from build123d import *

# Parameters (mm, degrees)
F0_R      = 8.89
F1_DEPTH  = 12.7
F2_R      = 6.35
F3_DEPTH  = 27.94
F5_DEPTH  = 43.18
F6_R      = 20.2522571076
F6_R_2    = 6.3246
F7_DEPTH  = 43.18
F8_R      = 4
F9_DEPTH  = 33.02
F13_D     = 2.2606
F13_DEPTH = 8.89
F13_START = 0.0721476
F13_TIP   = 0.6791527577
F14_R     = 8.89
F14_R_2   = 3.175
F15_DEPTH = 11.43


with BuildPart() as f1:
    # F0 (on Top) → F1 (new body)
    with BuildSketch(Plane.XY):
        Circle(F0_R)
    extrude(amount=F1_DEPTH)

    # F2 (on face) → F3 (join)
    with BuildSketch(Plane.XY.offset(12.7)):
        Circle(F2_R)
    extrude(amount=F3_DEPTH)

    # F4 (on face) → F5 (join)
    with BuildSketch(Plane.XY.offset(40.64)):
        Polygon((0, -10.668), (9.2387590076, 5.334), (-9.2387590076, 5.334), align=None)
    extrude(amount=F5_DEPTH)

    # F6 (on face) → F7 (cut, through all)
    with BuildSketch(Plane.XY.offset(83.82)):
        Circle(F6_R)
        Circle(F6_R_2, mode=Mode.SUBTRACT)
    extrude(amount=-F7_DEPTH, mode=Mode.SUBTRACT)

    # F8 (on face) → F9 (cut)
    with BuildSketch(Plane(origin=(0, 0, 0), x_dir=(1, 0, 0), z_dir=(0, 0, -1))):
        Circle(F8_R)
    extrude(amount=-F9_DEPTH, mode=Mode.SUBTRACT)

    # F13
    # its depths count from where the whole tool has entered the part; down to there all is cleared
    with Locations(Plane(origin=(-8.89, 0, 0), x_dir=(0, 1, 0), z_dir=(-1, 0, 0)).offset(-F13_START)):
        with Locations((0, -7.62)):
            Hole(F13_D / 2, depth=F13_DEPTH)
            with Locations((0, 0, -(F13_DEPTH + F13_TIP / 2))):  # 118° drill point
                Cone(0, F13_D / 2, F13_TIP, mode=Mode.SUBTRACT)

    # F14 (on face) → F15 (cut)
    with BuildSketch(Plane.XY.offset(83.82)):
        Circle(F14_R)
        Circle(F14_R_2, mode=Mode.SUBTRACT)
    extrude(amount=-F15_DEPTH, mode=Mode.SUBTRACT)


solid = f1.part
Source: CAD feature listing. Evaluate the final solid. Frame: model axes, mm. A direction names the side the tool comes from. Give positions to 0.01 mm unless a question says otherwise; leave off trailing zeros. Order: outer loops, then holes, each group sorted by start corner. A loop starts at its lowest first (then second) coordinate and runs counter-clockwise, first axis right, second up. Notation, with made-up numbers: (49.5, -16.75) -> (89.5, -16.75) arc R13 ccw to (89.5, 3.25) -> close; hole circle Ø3 at (-2, 75.5). An arc over 180 degrees is marked (long way). Use a Markdown table: item, result.
1) Contact query for flat-ended pins moving along their axis: P1, Ø2.5, axis at x = -1.5, y = -0.5, coming from the -Z side; P2, Ø1.5, axis at y = 2.5, z = 74, coming from the -X side; P3, Ø1.5, axis at y = -5, z = 61, coming from the -X side. Output: stop coordinate, or through.
Answer list:
| item | result |
|---|---|
| P1 | z = 33.02 |
| P2 | x = -2.65 |
| P3 | x = -3.71 |
2) Section query D-D, the plane z = 7.62. Return the cut outline in (x, y).
Answer list:
| item | result |
|---|---|
| outline | (-8.82, -1.13) arc R8.89 ccw (long way) to (-8.82, 1.13) -> (-3.84, 1.13) arc R4 cw (long way) to (-3.84, -1.13) -> close |
3) Section query B-B, the plane x = -5.25. Return the cut outline in (y, z), then the cut area to 3 significant figures.
Answer list:
| item | result |
|---|---|
| outline | (-7.17, 0) -> (7.17, 0) -> (7.17, 12.7) -> (3.57, 12.7) -> (3.57, 40.64) -> (3.53, 40.64) -> (3.53, 72.39) -> (-1.57, 72.39) -> (-1.57, 40.64) -> (-3.57, 40.64) -> (-3.57, 12.7) -> (-7.17, 12.7) -> close; hole circle Ø2.26 at (0, 7.62) |
| area | 540 mm² |
4) Reachability of faces 5 (the cylindrical face through (5.498, 3.125, 56.737)), 6 (the flat face through (-4.64, -2.63, 56.29)), 7 (the flat face through (0, 5.334, 56)) from +Z, -Z, +X, -X, +Y, -Y: full face, straight path, thin tool, end or side. Return the list, or none.
Answer list:
| item | result |
|---|---|
| face 5 | +Z, +X, +Y |
| face 6 | +Z, -X, -Y |
| face 7 | +Z, +X, -X, +Y |
5) Mould query, pull axis Y, two halves, no side actions, for faces 1 (the cylindrical face through (-5.456, 3.199, 56.737)), 2 (the cylindrical face through (-0.867, 3.905, 16.279)), 3 (the cylindrical face through (-0.69, -3.1, 78.19)), 4 (the flat face through (2, -4, 0)). Classes: +Y half, -Y half, draft (parallel to the pull), parting line (faces both ways), or undercut.
Answer list:
| item | result |
|---|---|
| face 1 | +Y half |
| face 2 | undercut |
| face 3 | parting line |
| face 4 | draft |
6) Ray query, line 1 along Y through (x, z) = (0, 10); line 2 along Y through (x, z) = (0, 19.5). Return the intervals inside material, ascending. Write a range as [from, to].
Answer list:
| item | result |
|---|---|
| line 1 | [-8.89, -4], [4, 8.89] |
| line 2 | [-6.35, -4], [4, 6.35] |
7) Section query A-A, the plane z = 46. Return the cut outline in (x, y).
Answer list:
| item | result |
|---|---|
| outline | (-6.32, 0.28) -> (-2.92, -5.61) arc R6.32 ccw to (2.92, -5.61) -> (6.32, 0.28) arc R6.32 ccw to (3.4, 5.33) -> (-3.4, 5.33) arc R6.32 ccw to start |
8) Section query C-C, the plane y = -7.25. Return the cut outline in (x, z), then the cut area to 3 significant figures.
Answer list:
| item | result |
|---|---|
| outline | (-5.14, 0) -> (5.14, 0) -> (5.14, 12.7) -> (-5.14, 12.7) -> close |
| area | 131 mm² |
